Build history of the part. All positions in model axes, mm. Face numbers are marked on the shaded views. A direction names the side the tool comes from. Round coordinates to 2 decimals unless told otherwise and drop trailing zeros. Loops run counter-clockwise (first coordinate to the right, second up) from the corner with the lowest first, then second, coordinate; pieces in that order, holes last. Notation, with made-up numbers: (-12.75, 53.25) - (9.25, 53.25) arc R21 ccw to (9.25, 71.25) - close; hole circle Ø11 at (26, 87). An arc over 180 degrees is marked (long way). Use a Markdown table: item, result.
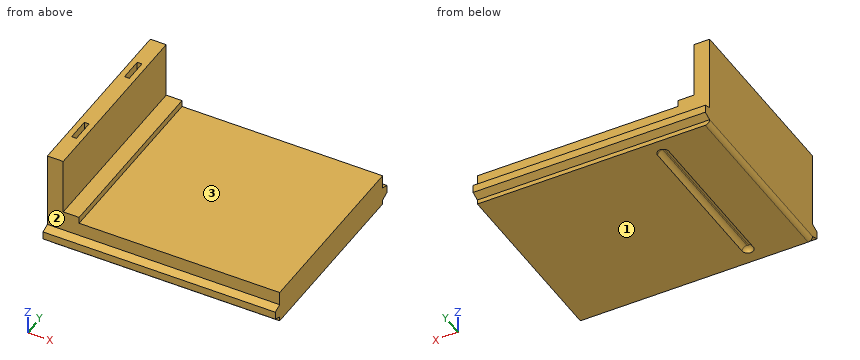
from build123d import *

# Parameters (mm, degrees)
F0_W         = 102.5
F0_H         = 82.3
F1_DEPTH     = 14
F2_W         = 7
F2_H         = 82.3
F3_DEPTH     = 27.9
F4_W         = 7
F4_H         = 82.3
F5_DEPTH     = 2.9
F7_DEPTH     = 102.5
F8_R         = 2
F11_DEPTH    = 2
F12_T1_DEPTH = 67.5
F12_T4_ANGLE = 180
F12_T6_ANGLE = 180
F13_W        = 2.1
F13_H        = 10.1
F14_DEPTH    = 19.95
F15_R        = 5.04999
F16_R        = 5.04999


# Not quite as in the source:
# - a fillet or chamfer that OpenCascade refuses, or shapes differently, is made with other operations: its cross-section is extruded or revolved along the edge and cut away or added
# - a fillet or chamfer is up to 0.001 mm smaller than in the source, because OpenCascade refuses the exact size


with BuildPart() as f1:
    # F0 (on Top) → F1 (new body)
    with BuildSketch(Plane.XY):
        Rectangle(F0_W, F0_H)
    extrude(amount=F1_DEPTH)

    # F2 (on face) → F3 (join)
    with BuildSketch(Plane.XY.offset(14)):
        with Locations((-47.75, 0)):
            Rectangle(F2_W, F2_H)
    extrude(amount=F3_DEPTH)

    # F4 (on face) → F5 (join)
    with BuildSketch(Plane.XY.offset(14)):
        with Locations((-40.75, 0)):
            Rectangle(F4_W, F4_H)
    extrude(amount=F5_DEPTH)

    # F6 (on face) → F7 (join)
    with BuildSketch(Plane.YZ.offset(51.25)):
        Polygon((41.15, 8), (41.15, 2), (44.65, 3.2738958199), (44.65, 6.7261041801), align=None)
        Polygon((-44.65, 3.2738958199), (-41.15, 2), (-41.15, 8), (-44.65, 6.7261041801), align=None)
    extrude(amount=-F7_DEPTH)

    # F8
    f8_edges = [f1.edges().sort_by_distance(p)[0] for p in [
        (-51.25, 0, 0),
    ]]
    fillet(f8_edges, radius=F8_R)

    # F10: union 

    # F9 (on face) → F11 (cut)
    with BuildSketch(Plane(origin=(0, 0, 0), x_dir=(1, 0, 0), z_dir=(0, 0, -1))):
        with BuildLine():
            ThreePointArc((-24.25, 33.65), (-26.75, 36.15), (-29.25, 33.65))
            Line((-29.25, 33.65), (-29.25, -33.85))
            ThreePointArc((-29.25, -33.85), (-26.75, -36.35), (-24.25, -33.85))
            Line((-24.25, -33.85), (-24.25, 33.65))
        make_face()
    extrude(amount=-F11_DEPTH, mode=Mode.SUBTRACT)

    # F12: fillet of radius 2.2 on 2 edges, made by hand

    # F12_s2 → F12_t1 (join)
    with BuildSketch(Plane.XZ.offset(-33.85)):
        with BuildLine():
            ThreePointArc((-29.25, 0), (-28.5423494674, 1.4248076809), (-27.05910977, 2))
            Line((-27.05910977, 2), (-29.25, 2))
            Line((-29.25, 2), (-29.25, 0))
        make_face()
        with BuildLine():
            ThreePointArc((-24.25, 0), (-24.9576505326, 1.4248076809), (-26.44089023, 2))
            Line((-26.44089023, 2), (-24.25, 2))
            Line((-24.25, 2), (-24.25, 0))
        make_face()
    extrude(amount=F12_T1_DEPTH)

    # F12_s3 → F12_t4 (revolve)
    with BuildSketch(Plane.XZ.offset(-33.85)):
        with BuildLine():
            ThreePointArc((-29.25, 0), (-28.5423494674, 1.4248076809), (-27.05910977, 2))
            Line((-27.05910977, 2), (-29.25, 2))
            Line((-29.25, 2), (-29.25, 0))
        make_face()
    revolve(axis=Axis((-26.75, 33.85, 2), (0, 0, -1)), revolution_arc=F12_T4_ANGLE)

    # F12_s5 → F12_t6 (revolve)
    with BuildSketch(Plane.XZ.offset(33.65)):
        with BuildLine():
            ThreePointArc((-24.25, 0), (-24.9576505326, 1.4248076809), (-26.44089023, 2))
            Line((-26.44089023, 2), (-24.25, 2))
            Line((-24.25, 2), (-24.25, 0))
        make_face()
    revolve(axis=Axis((-26.75, -33.65, 2), (0, 0, -1)), revolution_arc=F12_T6_ANGLE)

    # F13 (on face) → F14 (cut)
    with BuildSketch(Plane.XY.offset(41.9)):
        with Locations((-47.75, 21.15)):
            Rectangle(F13_W, F13_H)
        with Locations((-47.75, -21.15)):
            Rectangle(F13_W, F13_H)
    extrude(amount=-F14_DEPTH, mode=Mode.SUBTRACT)

    # F15 (radius 5.05 in the source; OpenCascade refuses exactly that, so slightly less here)
    f15_edges = [f1.edges().sort_by_distance(p)[0] for p in [
        (-47.75, 16.1, 21.95),
        (-47.75, 26.2, 21.95),
    ]]
    fillet(f15_edges, radius=F15_R)

    # F16 (radius 5.05 in the source; OpenCascade refuses exactly that, so slightly less here)
    f16_edges = [f1.edges().sort_by_distance(p)[0] for p in [
        (-47.75, -16.1, 21.95),
        (-47.75, -26.2, 21.95),
    ]]
    fillet(f16_edges, radius=F16_R)


solid = f1.part
Q1. Cut at D-D, the plane z = 11. List the corners of the cut face in (x, y), plus the area to 3 significant figures.
Results found:
| item | result |
|---|---|
| outline | (-51.25, -41.15) - (51.25, -41.15) - (51.25, 41.15) - (-51.25, 41.15) - close |
| area | 8,440 mm2 |
Q2. Cut at A-A, the plane z = 31.5. List the corners of the cut face in (x, y), plus the area to 3 significant figures.
Results found:
| item | result |
|---|---|
| outline | (-51.25, -41.15) - (-44.25, -41.15) - (-44.25, 41.15) - (-51.25, 41.15) - close; hole (-48.8, -26.2) - (-46.7, -26.2) - (-46.7, -16.1) - (-48.8, -16.1) - close; hole (-48.8, 16.1) - (-46.7, 16.1) - (-46.7, 26.2) - (-48.8, 26.2) - close |
| area | 534 mm2 |
Q3. Drop flat-ended pins along their axis: pin 1 (3 mm diameter, centred on x = 38.5, z = 11, fed in from -Y); pin 2 (6 mm diameter, centred on y = 28.5, z = 37.5, fed in from +X); pin 3 (5 mm diameter, centred on x = 25.5, y = -32, fed in from +Z). Give the stop position or say it passes through.
Results found:
| item | result |
|---|---|
| pin 1 | stops at y = -41.15 |
| pin 2 | stops at x = -44.25 |
| pin 3 | stops at z = 14 |
Q4. Cut at C-C, the plane x = 40.5. List the corners of the cut face in (y, z).
Results found:
| item | result |
|---|---|
| outline | (-44.65, 3.27) - (-41.15, 2) - (-41.15, 0) - (41.15, 0) - (41.15, 2) - (44.65, 3.27) - (44.65, 6.73) - (41.15, 8) - (41.15, 14) - (-41.15, 14) - (-41.15, 8) - (-44.65, 6.73) - close |
Q5. Probe line 1 (Z direction, x = -44, y = 31); line 2 (X direction, y = -18.5, z = 24); line 3 (X direction, y = 8.5, z = 32.5). List the from-to ranges inside material, lowest first.
Results found:
| item | result |
|---|---|
| line 1 | z = 0 to 16.9 |
| line 2 | x = -51.25 to -48.8, -46.7 to -44.25 |
| line 3 | x = -51.25 to -44.25 |
Q6. Cut at B-B, the plane y = -4. List the corners of the cut face in (x, z).
Results found:
| item | result |
|---|---|
| outline | (-51.25, 2) arc R2 ccw to (-49.25, 0) - (-29.25, 0) arc R2.2 cw to (-27.06, 2) - (-26.44, 2) arc R2.2 cw to (-24.25, 0) - (51.25, 0) - (51.25, 14) - (-37.25, 14) - (-37.25, 16.9) - (-44.25, 16.9) - (-44.25, 41.9) - (-51.25, 41.9) - close |
Q7. Which spindle directions (+Z, -Z, +X, -X, +Y, -Y) get a long thin tool onto all of the face, cutting with end or side? Do the marked faces 1, 2 and 3. Say none if no direction does.
Results found:
| item | result |
|---|---|
| face 1 | -Z, +X, -X, +Y, -Y |
| face 2 | +Z, +X, -X, -Y |
| face 3 | +Z, +X, +Y, -Y |
